Geometry: see drawing. Coordinates: mm, zero at the bounding-box minimum. A direction names the side the tool comes from. Coordinates: 2 decimals unless noted, no trailing zeros. Order: outer loops, then holes, each group sorted by start corner. A loop starts at its lowest first (then second) coordinate and runs counter-clockwise, first axis right, second up. Notation, with made-up numbers: (69, 86.5) -> (125, 86.5) arc R9 ccw to (125, 102.5) -> close; hole circle Ø9 at (-9.75, 3). An arc over 180 degrees is marked (long way). Use one line per item in the form item = value.
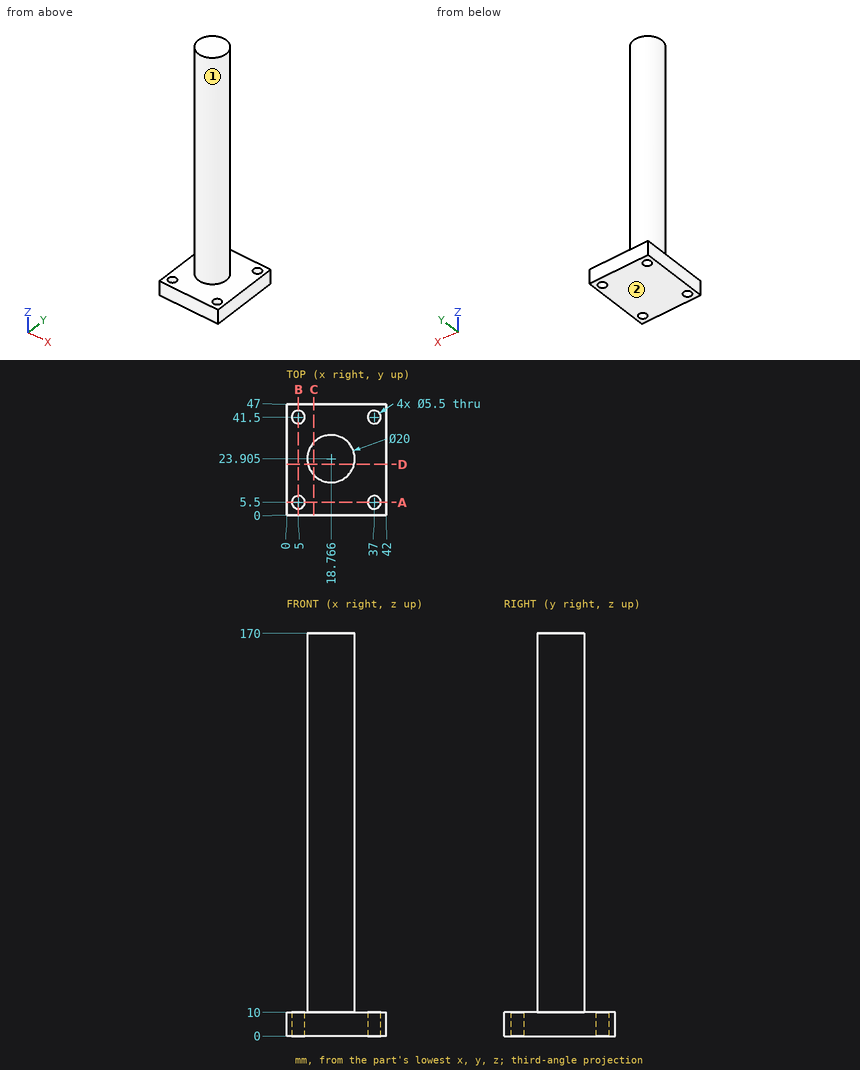
1) Material intervals for probe 1 along Y at (x, z) = (37, 7); probe 2 along X at (y, z) = (41, 2); probe 3 along Y at (x, z) = (18, 79.5), sorted ascending. Write a range as from..to.
Results found:
probe_1 = 0..2.75, 8.25..38.75, 44.25..47
probe_2 = 0..2.3, 7.7..34.3, 39.7..42
probe_3 = 13.93..33.88
2) Access query for the marked faces 1 and 2. Directions: +Z, -Z, +X, -X, +Y, -Y. A direction counts if a zero-diameter tool reaches every point of the face in a straight line with its end or side. Return the directions, or none.
Results found:
face_1 = +Z
face_2 = -Z, +X, -X, +Y, -Y
3) Section C-C, the plane x = 11.5. Output: boundary loops of the cut face in (y, z).
Results found:
outline = (0, 0) -> (47, 0) -> (47, 10) -> (30.78, 10) -> (30.78, 170) -> (17.03, 170) -> (17.03, 10) -> (0, 10) -> close
4) Section B-B, the plane x = 5. Output: boundary loops of the cut face in (y, z), and give its area (3 significant figures).
Results found:
outline = (0, 0) -> (2.75, 0) -> (2.75, 10) -> (0, 10) -> close; (8.25, 0) -> (38.75, 0) -> (38.75, 10) -> (8.25, 10) -> close; (44.25, 0) -> (47, 0) -> (47, 10) -> (44.25, 10) -> close
area = 360 mm2
5) Contact query for flat-ended pins moving along their axis: P1, Ø3.5, axis at x = 37, y = 5.5, coming from the +Z side; P2, Ø1, axis at x = 26.5, y = 35, coming from the +Z side; P3, Ø4, axis at y = 27, z = 55, coming from the +X side; P4, Ø10, axis at y = 29, z = 84.5, coming from the +X side. Output: stop coordinate, or through.
Results found:
P1 = through
P2 = 10
P3 = 28.71
P4 = 28.77
6) Section D-D, the plane y = 21.5. Output: boundary loops of the cut face in (x, z).
Results found:
outline = (0, 0) -> (42, 0) -> (42, 10) -> (28.47, 10) -> (28.47, 170) -> (9.06, 170) -> (9.06, 10) -> (0, 10) -> close
7) Section A-A, the plane y = 5.5. Output: boundary loops of the cut face in (x, z), and give its area (3 significant figures).
Results found:
outline = (0, 0) -> (2.25, 0) -> (2.25, 10) -> (0, 10) -> close; (7.75, 0) -> (34.25, 0) -> (34.25, 10) -> (7.75, 10) -> close; (39.75, 0) -> (42, 0) -> (42, 10) -> (39.75, 10) -> close
area = 310 mm2
